Geometry: see drawing. Coordinates: mm, zero at the bounding-box minimum. Round coordinates to 2 decimals unless told otherwise and drop trailing zeros. Write each loop counter-clockwise with the first axis right and the second up, starting at its lowest first coordinate (ties: lowest second). Pieces come first, ordered by that corner, then holes. Notation, with made-up numbers: M 86.5,26 L 130.5,26 A23 cw 130.5,52 Z; hole C 51,1 d7. An arc over 180 degrees is marked long. Write each question's results on one line, items separated by ' | '. Start each with the question number.
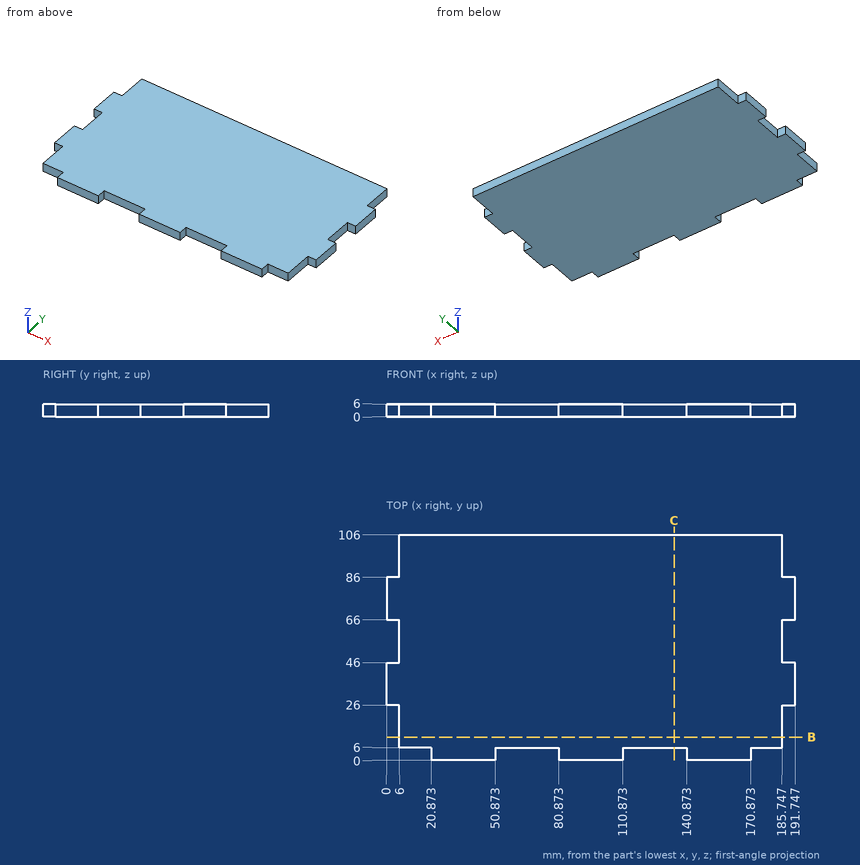
1. Cut plane C-C on x = 135. Output: boundary loops of the cut face in (y, z), and give its area (3 significant figures).
2. Contact query for flat-ended pins moving along their axis: P1, Ø1.8, axis at y = 4, z = 3, coming from the +X side; P2, Ø1.8, axis at x = 4, z = 3, coming from the -Y side; P3, Ø3, axis at x = 129, z = 3, coming from the -Y side. Output: stop coordinate, or through.
3. Line query: L1, parallel to X at y = 65.5, z = 4.6; L2, parallel to Y at x = 15.5, z = 1.7. Output: solid intervals per line, ascending. Write a range as from..to.
4. Cut plane B-B on y = 11. Output: boundary loops of the cut face in (x, z).
Answers follow:
1) outline: M 6,0 L 106,0 L 106,6 L 6,6 Z | area: 600 mm2
2) P1: stops at x = 170.87 | P2: stops at y = 26 | P3: stops at y = 6
3) L1: x = 6..185.75 | L2: y = 6..106
4) outline: M 6,0 L 185.75,0 L 185.75,6 L 6,6 Z
